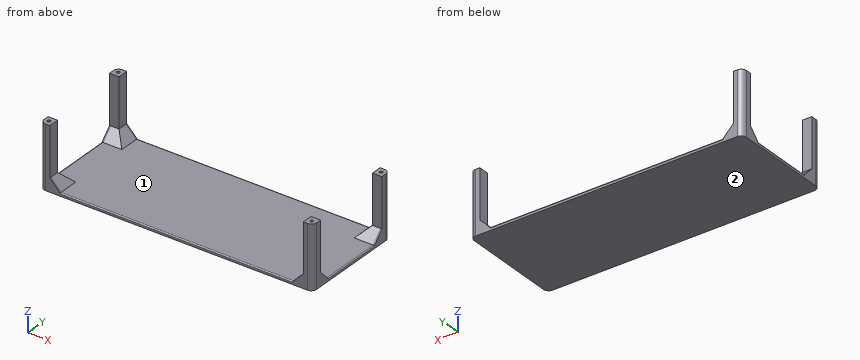
from build123d import *

# Parameters (mm, degrees)
SKETCH_1_W          = 260
SKETCH_1_H          = 100
EXTRUDE_1_DEPTH     = 3
SKETCH_2_W          = 9
SKETCH_2_H          = 10
EXTRUDE_2_DEPTH     = 60
FILLET_3_R          = 5
FILLET_4_R          = 1
SKETCH_3_R          = 1.5
CUT_EXTRUDE_1_DEPTH = 10
CHAMFER_1_SIZE      = 10


with BuildPart() as part:
    # 草图1 → 凸台-拉伸1 (new body)
    with BuildSketch(Plane.XY):
        Rectangle(SKETCH_1_W, SKETCH_1_H)
    extrude(amount=EXTRUDE_1_DEPTH)

    # 草图2 → 凸台-拉伸2 (add)
    with BuildSketch(Plane(origin=(0, 0, 0), x_dir=(-1, 0, 0), z_dir=(0, 0, -1))):
        with Locations((125.5, 45)):
            Rectangle(SKETCH_2_W, SKETCH_2_H)
        with Locations((125.5, -45)):
            Rectangle(SKETCH_2_W, SKETCH_2_H)
        with Locations((-125.5, -45)):
            Rectangle(SKETCH_2_W, SKETCH_2_H)
        with Locations((-125.5, 45)):
            Rectangle(SKETCH_2_W, SKETCH_2_H)
    extrude(amount=-EXTRUDE_2_DEPTH)

    # 圆角3
    fillet_3_edges = [part.edges().sort_by_distance(p)[0] for p in [
        (130, -50, 30),
        (-130, -50, 30),
        (-130, 50, 30),
        (130, 50, 30),
    ]]
    fillet(fillet_3_edges, radius=FILLET_3_R)

    # 圆角4
    fillet_4_edges = [part.edges().sort_by_distance(p)[0] for p in [
        (0, -50, 3),
        (-130, 0, 3),
        (130, 0, 3),
        (0, 50, 3),
    ]]
    fillet(fillet_4_edges, radius=FILLET_4_R)

    # 草图3 → 切除-拉伸1 (cut)
    with BuildSketch(Plane.XY.offset(60)):
        with Locations((125.5, -45)):
            Circle(SKETCH_3_R)
        with Locations((125.5, 45)):
            Circle(SKETCH_3_R)
        with Locations((-125.5, -45)):
            Circle(SKETCH_3_R)
        with Locations((-125.5, 45)):
            Circle(SKETCH_3_R)
    extrude(amount=-CUT_EXTRUDE_1_DEPTH, mode=Mode.SUBTRACT)

    # 倒角1
    # the kernel refuses this chamfer: 10 mm, written as the material it adds along each edge
    with BuildSketch(Plane(origin=(121, 40, 3), x_dir=(0, -1, 0), z_dir=(1, 0, 0))) as chamfer_1_piece_1:
        Polygon((CHAMFER_1_SIZE, 0), (0, -CHAMFER_1_SIZE), (0, 0), align=None)
    extrude(amount=8)
    with BuildSketch(Plane(origin=(-121, 49, 3), x_dir=(1, 0, 0), z_dir=(0, -1, 0))) as chamfer_1_piece_2:
        Polygon((CHAMFER_1_SIZE, 0), (0, CHAMFER_1_SIZE), (0, 0), align=None)
    extrude(amount=9)
    with BuildSketch(Plane(origin=(-129, -40, 3), x_dir=(0, 1, 0), z_dir=(1, 0, 0)), Plane(origin=(-121, 40, 3), x_dir=(0, -1, 0), z_dir=(-1, 0, 0)), Plane(origin=(121, -40, 3), x_dir=(0, 1, 0), z_dir=(1, 0, 0))) as chamfer_1_piece_3:
        Polygon((CHAMFER_1_SIZE, 0), (0, CHAMFER_1_SIZE), (0, 0), align=None)
    extrude(amount=8)
    with BuildSketch(Plane(origin=(121, -49, 3), x_dir=(0, 0, 1), z_dir=(0, 1, 0)), Plane(origin=(-121, -40, 3), x_dir=(0, 0, 1), z_dir=(0, -1, 0)), Plane(origin=(121, 49, 3), x_dir=(-1, 0, 0), z_dir=(0, -1, 0))) as chamfer_1_piece_4:
        Polygon((CHAMFER_1_SIZE, 0), (0, -CHAMFER_1_SIZE), (0, 0), align=None)
    extrude(amount=9)
    with BuildSketch(Plane(origin=(-121, 49, 2), x_dir=(0, 0, 1), z_dir=(0, -1, 0))) as chamfer_1_piece_5_section:
        Polygon((1 + CHAMFER_1_SIZE, 0), (1, -CHAMFER_1_SIZE), (1, 0), align=None)
    chamfer_1_piece_5 = revolve(axis=Axis((-121, 49, 2), (-1, 0, 0)), revolution_arc=359.64, mode=Mode.PRIVATE)
    chamfer_1_piece_5 = split(chamfer_1_piece_5, bisect_by=Plane(origin=(-121, 49, 0), z_dir=(0, 0, 1)), keep=Keep.TOP, mode=Mode.PRIVATE)
    chamfer_1_piece_5 = split(chamfer_1_piece_5, bisect_by=Plane(origin=(-121, 50, 2), z_dir=(0, -1, 0)), keep=Keep.TOP, mode=Mode.PRIVATE)
    add(chamfer_1_piece_5)
    with BuildSketch(Plane(origin=(121, 49, 2), x_dir=(0, 0, 1), z_dir=(0, -1, 0))) as chamfer_1_piece_6_section:
        Polygon((1, CHAMFER_1_SIZE), (1 + CHAMFER_1_SIZE, 0), (1, 0), align=None)
    chamfer_1_piece_6 = revolve(axis=Axis((121, 49, 2), (-1, 0, 0)), revolution_arc=359.64, mode=Mode.PRIVATE)
    chamfer_1_piece_6 = split(chamfer_1_piece_6, bisect_by=Plane(origin=(121, 49, 0), z_dir=(0, 0, 1)), keep=Keep.TOP, mode=Mode.PRIVATE)
    chamfer_1_piece_6 = split(chamfer_1_piece_6, bisect_by=Plane(origin=(121, 50, 2), z_dir=(0, -1, 0)), keep=Keep.TOP, mode=Mode.PRIVATE)
    add(chamfer_1_piece_6)
    with BuildSketch(Plane(origin=(-129, -40, 2), x_dir=(0, 0, 1), z_dir=(1, 0, 0))) as chamfer_1_piece_7_section:
        Polygon((1 + CHAMFER_1_SIZE, 0), (1, -CHAMFER_1_SIZE), (1, 0), align=None)
    chamfer_1_piece_7 = revolve(axis=Axis((-129, -40, 2), (0, -1, 0)), revolution_arc=359.64, mode=Mode.PRIVATE)
    chamfer_1_piece_7 = split(chamfer_1_piece_7, bisect_by=Plane(origin=(-129, -40, 0), z_dir=(0, 0, 1)), keep=Keep.TOP, mode=Mode.PRIVATE)
    chamfer_1_piece_7 = split(chamfer_1_piece_7, bisect_by=Plane(origin=(-130, -40, 2), z_dir=(1, 0, 0)), keep=Keep.TOP, mode=Mode.PRIVATE)
    add(chamfer_1_piece_7)
    with BuildSketch(Plane(origin=(-129, 40, 2), x_dir=(0, 0, 1), z_dir=(1, 0, 0))) as chamfer_1_piece_8_section:
        Polygon((1, CHAMFER_1_SIZE), (1 + CHAMFER_1_SIZE, 0), (1, 0), align=None)
    chamfer_1_piece_8 = revolve(axis=Axis((-129, 40, 2), (0, -1, 0)), revolution_arc=359.64, mode=Mode.PRIVATE)
    chamfer_1_piece_8 = split(chamfer_1_piece_8, bisect_by=Plane(origin=(-129, 40, 0), z_dir=(0, 0, 1)), keep=Keep.TOP, mode=Mode.PRIVATE)
    chamfer_1_piece_8 = split(chamfer_1_piece_8, bisect_by=Plane(origin=(-130, 40, 2), z_dir=(1, 0, 0)), keep=Keep.TOP, mode=Mode.PRIVATE)
    add(chamfer_1_piece_8)
    with BuildSketch(Plane(origin=(129, 40, 2), x_dir=(0, 0, 1), z_dir=(-1, 0, 0))) as chamfer_1_piece_9_section:
        Polygon((1, -CHAMFER_1_SIZE), (1 + CHAMFER_1_SIZE, 0), (1, 0), align=None)
    chamfer_1_piece_9 = revolve(axis=Axis((129, 40, 2), (0, 1, 0)), revolution_arc=359.64, mode=Mode.PRIVATE)
    chamfer_1_piece_9 = split(chamfer_1_piece_9, bisect_by=Plane(origin=(129, 40, 0), z_dir=(0, 0, 1)), keep=Keep.TOP, mode=Mode.PRIVATE)
    chamfer_1_piece_9 = split(chamfer_1_piece_9, bisect_by=Plane(origin=(130, 40, 2), z_dir=(-1, 0, 0)), keep=Keep.TOP, mode=Mode.PRIVATE)
    add(chamfer_1_piece_9)
    with BuildSketch(Plane(origin=(129, -40, 2), x_dir=(0, 0, 1), z_dir=(-1, 0, 0))) as chamfer_1_piece_10_section:
        Polygon((1 + CHAMFER_1_SIZE, 0), (1, CHAMFER_1_SIZE), (1, 0), align=None)
    chamfer_1_piece_10 = revolve(axis=Axis((129, -40, 2), (0, 1, 0)), revolution_arc=359.64, mode=Mode.PRIVATE)
    chamfer_1_piece_10 = split(chamfer_1_piece_10, bisect_by=Plane(origin=(129, -40, 0), z_dir=(0, 0, 1)), keep=Keep.TOP, mode=Mode.PRIVATE)
    chamfer_1_piece_10 = split(chamfer_1_piece_10, bisect_by=Plane(origin=(130, -40, 2), z_dir=(-1, 0, 0)), keep=Keep.TOP, mode=Mode.PRIVATE)
    add(chamfer_1_piece_10)
    with BuildSketch(Plane(origin=(121, -49, 2), x_dir=(0, 0.006283143965553963, 0.9999802608561372), z_dir=(0, -0.9999802608561372, 0.006283143965553963))) as chamfer_1_piece_11_section:
        Polygon((1, CHAMFER_1_SIZE), (1 + CHAMFER_1_SIZE, 0), (1, 0), align=None)
    chamfer_1_piece_11 = revolve(axis=Axis((121, -49, 2), (-1, 0, 0)), revolution_arc=359.64, mode=Mode.PRIVATE)
    chamfer_1_piece_11 = split(chamfer_1_piece_11, bisect_by=Plane(origin=(121, -50, 2), z_dir=(0, 1, 0)), keep=Keep.TOP, mode=Mode.PRIVATE)
    chamfer_1_piece_11 = split(chamfer_1_piece_11, bisect_by=Plane(origin=(121, -49, 0), z_dir=(0, 0, 1)), keep=Keep.TOP, mode=Mode.PRIVATE)
    add(chamfer_1_piece_11)
    with BuildSketch(Plane(origin=(-121, -49, 2), x_dir=(0, 0.006283143965553963, 0.9999802608561372), z_dir=(0, -0.9999802608561372, 0.006283143965553963))) as chamfer_1_piece_12_section:
        Polygon((1 + CHAMFER_1_SIZE, 0), (1, -CHAMFER_1_SIZE), (1, 0), align=None)
    chamfer_1_piece_12 = revolve(axis=Axis((-121, -49, 2), (-1, 0, 0)), revolution_arc=359.64, mode=Mode.PRIVATE)
    chamfer_1_piece_12 = split(chamfer_1_piece_12, bisect_by=Plane(origin=(-121, -50, 2), z_dir=(0, 1, 0)), keep=Keep.TOP, mode=Mode.PRIVATE)
    chamfer_1_piece_12 = split(chamfer_1_piece_12, bisect_by=Plane(origin=(-121, -49, 0), z_dir=(0, 0, 1)), keep=Keep.TOP, mode=Mode.PRIVATE)
    add(chamfer_1_piece_12)
    with BuildSketch(Plane(origin=(95.28317012, 40, 3), x_dir=(0, -1, 0), z_dir=(1, 0, 0))) as chamfer_1_piece_13a_section:
        Polygon((CHAMFER_1_SIZE, 0), (0, -CHAMFER_1_SIZE), (0, 0), align=None)
    chamfer_1_piece_13a = extrude(amount=33.71682988, mode=Mode.PRIVATE)
    chamfer_1_piece_13a = split(chamfer_1_piece_13a, bisect_by=Plane(origin=(121, 40, 3), z_dir=(-1, 0, 0)), keep=Keep.TOP, mode=Mode.PRIVATE)
    with BuildSketch(Plane(origin=(121, 49, 3), x_dir=(-1, 0, 0), z_dir=(0, -1, 0))) as chamfer_1_piece_13b_section:
        Polygon((CHAMFER_1_SIZE, 0), (0, -CHAMFER_1_SIZE), (0, 0), align=None)
    chamfer_1_piece_13b = extrude(amount=34.71682988, mode=Mode.PRIVATE)
    chamfer_1_piece_13b = split(chamfer_1_piece_13b, bisect_by=Plane(origin=(121, 40, 3), z_dir=(0, -1, 0)), keep=Keep.TOP, mode=Mode.PRIVATE)
    chamfer_1_piece_13 = chamfer_1_piece_13a & chamfer_1_piece_13b
    add(chamfer_1_piece_13)
    with BuildSketch(Plane(origin=(-95.28317012, 40, 3), x_dir=(0, -1, 0), z_dir=(-1, 0, 0))) as chamfer_1_piece_14a_section:
        Polygon((CHAMFER_1_SIZE, 0), (0, CHAMFER_1_SIZE), (0, 0), align=None)
    chamfer_1_piece_14a = extrude(amount=33.71682988, mode=Mode.PRIVATE)
    chamfer_1_piece_14a = split(chamfer_1_piece_14a, bisect_by=Plane(origin=(-121, 40, 3), z_dir=(1, 0, 0)), keep=Keep.TOP, mode=Mode.PRIVATE)
    with BuildSketch(Plane(origin=(-121, 49, 3), x_dir=(1, 0, 0), z_dir=(0, -1, 0))) as chamfer_1_piece_14b_section:
        Polygon((CHAMFER_1_SIZE, 0), (0, CHAMFER_1_SIZE), (0, 0), align=None)
    chamfer_1_piece_14b = extrude(amount=34.71682988, mode=Mode.PRIVATE)
    chamfer_1_piece_14b = split(chamfer_1_piece_14b, bisect_by=Plane(origin=(-121, 40, 3), z_dir=(0, -1, 0)), keep=Keep.TOP, mode=Mode.PRIVATE)
    chamfer_1_piece_14 = chamfer_1_piece_14a & chamfer_1_piece_14b
    add(chamfer_1_piece_14)
    with BuildSketch(Plane(origin=(-121, -14.28317012, 3), x_dir=(0, 0, 1), z_dir=(0, -1, 0))) as chamfer_1_piece_15a_section:
        Polygon((CHAMFER_1_SIZE, 0), (0, -CHAMFER_1_SIZE), (0, 0), align=None)
    chamfer_1_piece_15a = extrude(amount=34.71682988, mode=Mode.PRIVATE)
    chamfer_1_piece_15a = split(chamfer_1_piece_15a, bisect_by=Plane(origin=(-121, -40, 3), z_dir=(0, 1, 0)), keep=Keep.TOP, mode=Mode.PRIVATE)
    with BuildSketch(Plane(origin=(-129, -40, 3), x_dir=(0, 1, 0), z_dir=(1, 0, 0))) as chamfer_1_piece_15b_section:
        Polygon((CHAMFER_1_SIZE, 0), (0, CHAMFER_1_SIZE), (0, 0), align=None)
    chamfer_1_piece_15b = extrude(amount=33.71682988, mode=Mode.PRIVATE)
    chamfer_1_piece_15b = split(chamfer_1_piece_15b, bisect_by=Plane(origin=(-121, -40, 3), z_dir=(1, 0, 0)), keep=Keep.TOP, mode=Mode.PRIVATE)
    chamfer_1_piece_15 = chamfer_1_piece_15a & chamfer_1_piece_15b
    add(chamfer_1_piece_15)
    with BuildSketch(Plane(origin=(121, -49, 3), x_dir=(0, 0, 1), z_dir=(0, 1, 0))) as chamfer_1_piece_16a_section:
        Polygon((CHAMFER_1_SIZE, 0), (0, -CHAMFER_1_SIZE), (0, 0), align=None)
    chamfer_1_piece_16a = extrude(amount=34.71682988, mode=Mode.PRIVATE)
    chamfer_1_piece_16a = split(chamfer_1_piece_16a, bisect_by=Plane(origin=(121, -40, 3), z_dir=(0, 1, 0)), keep=Keep.TOP, mode=Mode.PRIVATE)
    with BuildSketch(Plane(origin=(95.28317012, -40, 3), x_dir=(0, 1, 0), z_dir=(1, 0, 0))) as chamfer_1_piece_16b_section:
        Polygon((CHAMFER_1_SIZE, 0), (0, CHAMFER_1_SIZE), (0, 0), align=None)
    chamfer_1_piece_16b = extrude(amount=33.71682988, mode=Mode.PRIVATE)
    chamfer_1_piece_16b = split(chamfer_1_piece_16b, bisect_by=Plane(origin=(121, -40, 3), z_dir=(-1, 0, 0)), keep=Keep.TOP, mode=Mode.PRIVATE)
    chamfer_1_piece_16 = chamfer_1_piece_16a & chamfer_1_piece_16b
    add(chamfer_1_piece_16)


solid = part.part
Could you check a few things on this model? Use its own coordinates, in mm. Face numbers are marked on the shaded views. Coordinates: 2 decimals unless noted, no trailing zeros. Write each loop counter-clockwise with the first axis right and the second up, starting at its lowest first coordinate (ties: lowest second). Pieces come first, ordered by that corner, then holes. Notation, with made-up numbers: (40.25, 71) - (44.25, 71) arc R29 ccw to (44.25, 109) - close; hole circle Ø10 at (56, -29). An arc over 180 degrees is marked (long way). Put each result on its own line as item: value. Start each with the question number.
Q1. I'm going to push flat-ended pins straight in: P1, Ø2, axis at x = -23.5, y = -18.5, coming from the +Z side; P2, Ø1.8, axis at x = -125.5, y = -45, coming from the +Z side; P3, Ø2.5, axis at x = 127, z = 45, coming from the -Y side. Where does each tip first touch, or does it pass through?
Q2. Please list where these lines run through material, in increasing order: L1, parallel to Y at x = -125.5, z = 57.25; L2, parallel to Y at x = -125, z = 58; L3, parallel to X at y = 45, z = 44.
Q3. Thinking about a two-plate mould opening in Z: for the marked faces 1 and 2, which applies, pulls with the +Z half, pulls with the -Z half, needs draft (parallel to the pull), parting line crosses it, or undercut?
Q4. I want a section at B-B on x = -36. Write out the boundary of the cut face in (y, z).
Q5. I want a section at C-C on y = -17.5. Write out the boundary of the cut face in (x, z), plus the area to 3 significant figures.
Q6. I want a section at A-A on z = 56. Write out the boundary of the cut face in (x, y).
Checks:
1. P1: z = 3
1. P2: z = 50
1. P3: y = -49.94
2. L1: -49.97 to -46.5, -43.5 to -40, 40 to 43.5, 46.5 to 49.97
2. L2: -50 to -46.41, -43.59 to -40, 40 to 43.59, 46.41 to 50
2. L3: -130 to -121, 121 to 130
3. face 1: pulls with the +Z half
3. face 2: pulls with the -Z half
4. outline: (-50, 0) - (50, 0) - (50, 2) arc R1 ccw to (49, 3) - (-49, 3) arc R1 ccw to (-50, 2) - close
5. outline: (-130, 0) - (130, 0) - (130, 2) arc R1 ccw to (129, 3) - (-129, 3) arc R1 ccw to (-130, 2) - close
5. area: 780 mm²
6. outline: (-130, -45) arc R5 ccw to (-125, -50) - (-121, -50) - (-121, -40) - (-130, -40) - close; (-130, 40) - (-121, 40) - (-121, 50) - (-125, 50) arc R5 ccw to (-130, 45) - close; (121, -50) - (125, -50) arc R5 ccw to (130, -45) - (130, -40) - (121, -40) - close; (121, 40) - (130, 40) - (130, 45) arc R5 ccw to (125, 50) - (121, 50) - close; hole circle Ø3 at (-125.5, -45); hole circle Ø3 at (-125.5, 45); hole circle Ø3 at (125.5, -45); hole circle Ø3 at (125.5, 45)
